Here's how the part is built. I have some questions about the finished solid (model axes, mm). A direction names the side the tool comes from. Round coordinates to 2 decimals unless told otherwise and drop trailing zeros. Order: outer loops, then holes, each group sorted by start corner. A loop starts at its lowest first (then second) coordinate and runs counter-clockwise, first axis right, second up. Notation, with made-up numbers: (1, 66.5) -> (53, 66.5) arc R31 ccw to (53, 100.5) -> close; hole circle Ø11 at (33, -11.75). An arc over 180 degrees is marked (long way). One line per item, written item: value.
```python
from build123d import *

# Parameters (mm, degrees)
F1_DEPTH  = 10
F3_DEPTH  = 20
F4_R      = 1.3
F5_DEPTH  = 25
F4_R_2    = 4
F6_DEPTH  = 10
F8_R      = 1.3
F9_DEPTH  = 8
F7_R      = 1.3
F10_DEPTH = 8
F11_R     = 1.3
F12_DEPTH = 8


with BuildPart() as f1:
    # F0 (on Front) → F1 (new body, symmetric)
    with BuildSketch(Plane.XZ):
        Polygon((25.9807621135, -15), (25.9807621135, 15), (18.1865334795, 19.5), (15.1865334795, 14.3038475773), (20.3826859022, 11.3038475773), (17.3826859022, 6.1076951546), (-3.4019237886, 18.1076951546), (-0.4019237886, 23.3038475773), (7.3923048454, 18.8038475773), (10.3923048454, 24), (0, 30), (-25.9807621135, 15), (-25.9807621135, 6), (-19.9807621135, 6), (-19.9807621135, 12), (-13.9807621135, 12), (-13.9807621135, -12), (-19.9807621135, -12), (-19.9807621135, -3), (-25.9807621135, -3), (-25.9807621135, -15), (0, -30), (7.7942286341, -25.5), (4.7942286341, -20.3038475773), (-0.4019237886, -23.3038475773), (-3.4019237886, -18.1076951546), (17.3826859022, -6.1076951546), (20.3826859022, -11.3038475773), (12.5884572681, -15.8038475773), (15.5884572681, -21), align=None)
    extrude(amount=F1_DEPTH, both=True)

    # F2 (on face) → F3 (cut)
    with BuildSketch(Plane.XZ.offset(10)):
        with BuildLine():
            ThreePointArc((-2.9155494421, 1.3189281445), (-0.6746264837, -3.1280791402), (3.2, 0))
            ThreePointArc((3.2, 0), (2.3716827586, 2.1482832431), (0.3155494421, 3.1844039551))
            ThreePointArc((0.3155494421, 3.1844039551), (-1.6, 2.7712812921), (-2.9155494421, 1.3189281445))
        make_face()
        with BuildLine():
            ThreePointArc((-2.9155494421, 1.3189281445), (-1.6, 2.7712812921), (0.3155494421, 3.1844039551))
            Line((0.3155494421, 3.1844039551), (3.1670527423, 4.8307201531))
            Line((3.1670527423, 4.8307201531), (0.6670527423, 9.160847172))
            Line((0.6670527423, 9.160847172), (-7.9932012956, 4.160847172))
            Line((-7.9932012956, 4.160847172), (-5.4932012956, -0.1692798469))
            Line((-5.4932012956, -0.1692798469), (-2.9155494421, 1.3189281445))
        make_face()
    extrude(amount=-F3_DEPTH, mode=Mode.SUBTRACT)

    # F4 (on face) → F5 (cut)
    with BuildSketch(Plane(origin=(-12.9903810568, 0, 22.5), x_dir=(0.8660254038, 0, 0.5), z_dir=(-0.5, 0, 0.8660254038))):
        Circle(F4_R)
    extrude(amount=-F5_DEPTH, mode=Mode.SUBTRACT)

    # F4 (on face) → F6 (cut)
    with BuildSketch(Plane(origin=(-12.9903810568, 0, 22.5), x_dir=(0.8660254038, 0, 0.5), z_dir=(-0.5, 0, 0.8660254038))):
        Circle(F4_R_2)
        Circle(F4_R, mode=Mode.SUBTRACT)
    extrude(amount=-F6_DEPTH, mode=Mode.SUBTRACT)

    # F8 (on face) → F9 (cut)
    with BuildSketch(Plane(origin=(12.9903810568, 0, 22.5), x_dir=(0.8660254038, 0, -0.5), z_dir=(0.5, 0, 0.8660254038))):
        with Locations((-10, 0)):
            Circle(F8_R)
    extrude(amount=-F9_DEPTH, mode=Mode.SUBTRACT)

    # F7 (on face) → F10 (cut)
    with BuildSketch(Plane(origin=(12.9903810568, 0, -22.5), x_dir=(0.8660254038, 0, 0.5), z_dir=(0.5, 0, -0.8660254038))):
        with Locations((10, 0)):
            Circle(F7_R)
    extrude(amount=-F10_DEPTH, mode=Mode.SUBTRACT)

    # F11 (on face) → F12 (cut)
    with BuildSketch(Plane(origin=(-25.9807621135, 0, 0), x_dir=(0, -1, 0), z_dir=(-1, 0, 0))):
        with Locations((0, -10)):
            Circle(F11_R)
    extrude(amount=-F12_DEPTH, mode=Mode.SUBTRACT)


solid = f1.part
```
Q1. Which directions (+Z, -Z, +X, -X, +Y, -Y) give clear straight access to the entire face, cutting with the end or side of a thin tool? Please do faces 4 (the face through (-23, 0, -3)), 5 (the face through (-23.02, 0.17, -8.71)), 6 (the face through (-1.923, -0.14, 20.669)).
Answers:
face 4: -X, +Y, -Y
face 5: -X
face 6: +Y, -Y
Q2. I want a section at A-A on z = -2. Write out the boundary of the cut face in (x, y), then the cut area to 3 significant figures.
Answers:
outline: (-13.98, -10) -> (-2.5, -10) -> (-2.5, 10) -> (-13.98, 10) -> close; (2.5, -10) -> (25.98, -10) -> (25.98, 10) -> (2.5, 10) -> close
area: 699 mm2
Q3. I need wall thicknesses on line 1 along X through (y, z) = (-3.5, 0); line 2 along X through (y, z) = (1.5, -5); line 3 along Z through (x, y) = (0, 2.5). Which ranges of each line are inside material? Lowest first, please.
Answers:
line 1: -13.98 to -5.59, -5.2 to -3.2, 3.2 to 25.98
line 2: -25.98 to -19.98, -13.98 to 25.98
line 3: -30 to -23.07, -16.14 to -3.2, 8.78 to 16.14, 23.07 to 30
Q4. I want a section at B-B on x = -18. Write out the boundary of the cut face in (y, z), then the cut area to 3 significant figures.
Answers:
outline: (-10, -19.61) -> (10, -19.61) -> (10, -12) -> (-10, -12) -> close; (-10, 12) -> (10, 12) -> (10, 19.61) -> (-10, 19.61) -> close
area: 304 mm2
Q5. I want a section at D-D on z = -10. Write out the boundary of the cut face in (x, y).
Answers:
outline: (-25.98, -10) -> (-19.98, -10) -> (-19.98, -1.3) -> (-25.98, -1.3) -> close; (-25.98, 1.3) -> (-19.98, 1.3) -> (-19.98, 10) -> (-25.98, 10) -> close; (-13.98, -10) -> (10.64, -10) -> (10.64, 10) -> (-13.98, 10) -> close; (19.63, -10) -> (25.98, -10) -> (25.98, 10) -> (19.63, 10) -> close
Q6. I want a section at C-C on x = -1.5. Write out the boundary of the cut face in (y, z), then the cut area to 3 significant figures.
Answers:
outline: (-10, -29.13) -> (10, -29.13) -> (10, -21.4) -> (-10, -21.4) -> close; (-10, -17.01) -> (10, -17.01) -> (10, -2.83) -> (-10, -2.83) -> close; (-10, 7.91) -> (10, 7.91) -> (10, 17.01) -> (-10, 17.01) -> close; (-10, 21.4) -> (10, 21.4) -> (10, 29.13) -> (-10, 29.13) -> close
area: 775 mm2
Q7. For P1, Ø10, axis at x = 6.5, y = 6.5, coming from the +Z side; P2, Ø5, axis at x = -23, y = -2, coming from the -Z side; P3, Ø12, axis at y = -4.5, z = -16.5, coming from the +X side; P4, Ø5, axis at x = -16, y = -4.5, coming from the +Z side, each with a flat end and sliding along its axis, tell me the tip position at first contact or that it passes through.
Answers:
P1: z = 29.13
P2: z = -18.16
P3: x = 25.98
P4: z = 22.21
Q8. If we mould it in two halves opening along Z, with no side actions, what happens to faces 1 (the face through (-8.04, -1.72, 13.81)), 2 (the face through (-25.981, 0, -8)), 3 (the face through (16.71, -0.14, 16.94))? For each: pulls with the +Z half, pulls with the -Z half, needs draft (parallel to the pull), parting line crosses it, or undercut.
Answers:
face 1: undercut
face 2: needs draft
face 3: pulls with the +Z half
